The model under review builds one solid part; all positions refer to its coordinate system, in mm. A direction names the side the tool comes from. Give positions to 0.01 mm unless a question says otherwise; leave off trailing zeros. Order: outer loops, then holes, each group sorted by start corner. A loop starts at its lowest first (then second) coordinate and runs counter-clockwise, first axis right, second up. Notation, with made-up numbers: (-7, 58) -> (26, 58) arc R13 ccw to (26, 70) -> close; hole circle Ø11 at (-36.75, 58). An arc over 180 degrees is marked (long way). Use one line per item in the form item = value.
```python
from build123d import *

# Parameters (mm, degrees)
SKETCH1_W           = 25
SKETCH1_H           = 50
BOSS_EXTRUDE1_DEPTH = 30
SKETCH2_W           = 50
SKETCH2_H           = 8.605036789
BOSS_EXTRUDE2_DEPTH = 20
SKETCH3_R           = 4
CUT_EXTRUDE1_DEPTH  = 47.249264327
SKETCH4_W           = 10.2
SKETCH4_H           = 20.2
CUT_EXTRUDE2_DEPTH  = 20
BOSS_EXTRUDE3_DEPTH = 1


with BuildPart() as part:
    # Sketch1 → Boss-Extrude1 (new body)
    with BuildSketch(Plane(origin=(0, 0, 0), x_dir=(1, 0, 0), z_dir=(0, 1, 0))):
        Rectangle(SKETCH1_W, SKETCH1_H)
    extrude(amount=BOSS_EXTRUDE1_DEPTH)

    # Sketch2 → Boss-Extrude2 (add)
    with BuildSketch(Plane.ZY.offset(12.5)):
        with Locations((0, 4.302518394)):
            Rectangle(SKETCH2_W, SKETCH2_H)
    extrude(amount=BOSS_EXTRUDE2_DEPTH)

    # Sketch3 → Cut-Extrude1 (cut, through all)
    with BuildSketch(Plane(origin=(0, 8.605036789, 0), x_dir=(1, 0, 0), z_dir=(0, 1, 0))):
        with Locations(Location((-24.5, 15, 0), (0, 0, 270))):
            Circle(SKETCH3_R)
        with Locations(Location((-24.5, -15, 0), (0, 0, 270))):
            Circle(SKETCH3_R)
    extrude(amount=-CUT_EXTRUDE1_DEPTH, mode=Mode.SUBTRACT)

    # Sketch4 → Cut-Extrude2 (cut)
    with BuildSketch(Plane(origin=(12.5, 0, 0), x_dir=(0, 0, -1), z_dir=(1, 0, 0))):
        with Locations((-15, 15)):
            Rectangle(SKETCH4_W, SKETCH4_H)
    extrude(amount=-CUT_EXTRUDE2_DEPTH, mode=Mode.SUBTRACT)

    # Sketch5 → Boss-Extrude3 (add)
    with BuildSketch(Plane(origin=(0, 30, 0), x_dir=(1, 0, 0), z_dir=(0, 1, 0))):
        Polygon((-5.384615385, -10), (-5.384615385, 10), (-2.564102564, 10), (-2.564102564, -7.692307692), (6.923076923, -7.692307692), (6.923076923, -10), align=None)
    extrude(amount=BOSS_EXTRUDE3_DEPTH)


solid = part.part
```
1. Add section D-D on y = 3. Give the boundary of the cut face in (x, z), then the cut area to 3 significant figures.
Values:
outline = (-32.5, -25) -> (12.5, -25) -> (12.5, 25) -> (-32.5, 25) -> close; hole circle Ø8 at (-24.5, -15); hole circle Ø8 at (-24.5, 15)
area = 2,150 mm^2
2. Add section B-B on x = -1.5. Give the boundary of the cut face in (y, z).
Values:
outline = (0, -25) -> (30, -25) -> (30, 7.69) -> (31, 7.69) -> (31, 10) -> (30, 10) -> (30, 25) -> (0, 25) -> close; hole (4.9, 9.9) -> (25.1, 9.9) -> (25.1, 20.1) -> (4.9, 20.1) -> close
3. Add section C-C on x = -24.5. Give the boundary of the cut face in (y, z), then the cut area to 3 significant figures.
Values:
outline = (0, -25) -> (8.61, -25) -> (8.61, -19) -> (0, -19) -> close; (0, -11) -> (8.61, -11) -> (8.61, 11) -> (0, 11) -> close; (0, 19) -> (8.61, 19) -> (8.61, 25) -> (0, 25) -> close
area = 293 mm^2
4. Add section A-A on z = -15. Give the boundary of the cut face in (x, y).
Values:
outline = (-32.5, 0) -> (-28.5, 0) -> (-28.5, 8.61) -> (-32.5, 8.61) -> close; (-20.5, 0) -> (12.5, 0) -> (12.5, 30) -> (-12.5, 30) -> (-12.5, 8.61) -> (-20.5, 8.61) -> close
5. Tool access review of faces 1 (the face through (12.5, 15, 0)), 2 (the face through (-22, 8.605, 0)), 3 (the face through (3, 15, 9.9)): name each direction out of +Z, -Z, +X, -X, +Y, -Y from which nothing blocks a thin tool from reaching the whole face with its end or side.
Values:
face_1 = +Z, -Z, +X, +Y, -Y
face_2 = +Z, -Z, -X, +Y
face_3 = +X
6. For pin 1 Ø0.5 at (y, z) = (30.5, 9.5) entering from +X; pin 2 Ø10 at (y, z) = (22.5, -2.5) entering from -X; pin 3 Ø3 at (y, z) = (18.5, 17.5) entering from +X; pin 4 Ø8 at (x, z) = (0, 13) entering from +Y, all flat-tipped, find the tip position at first contact; note any pin that passes through.
Values:
pin_1 = 6.92
pin_2 = -12.5
pin_3 = -7.5
pin_4 = 31
7. For L1, parallel to Z at x = 0, y = 14.5; L2, parallel to Y at x = 1, z = 16.5; L3, parallel to X at y = 6.25, z = -15, list the stretches that pass through material, from the lowest coordinate up.
Values:
L1 = -25 to 9.9, 20.1 to 25
L2 = 0 to 4.9, 25.1 to 30
L3 = -32.5 to -28.5, -20.5 to 12.5
8. The part is to be moulded in two halves that separate along Y. For faces 4 (the face through (3, 4.9, 15)), 5 (the face through (-21.8, 4.36, 12.05)), 6 (the face through (-3, 31, 3)), say which applies: +Y half, -Y half, draft (parallel to the pull), parting line (faces both ways), or undercut.
Values:
face_4 = undercut
face_5 = draft
face_6 = +Y half
